Work out the finished part from the listing and answer in its coordinate system (mm). Face numbers are marked on the shaded views. A direction names the side the tool comes from. Coordinates: 2 decimals unless noted, no trailing zeros. Loops run counter-clockwise (first coordinate to the right, second up) from the corner with the lowest first, then second, coordinate; pieces in that order, holes last. Notation, with made-up numbers: (83.5, 13) -> (134.5, 13) arc R19 ccw to (134.5, 19) -> close; hole circle Ø8 at (58.5, -36). An arc over 180 degrees is marked (long way). One line per question, with ' | ' between items.
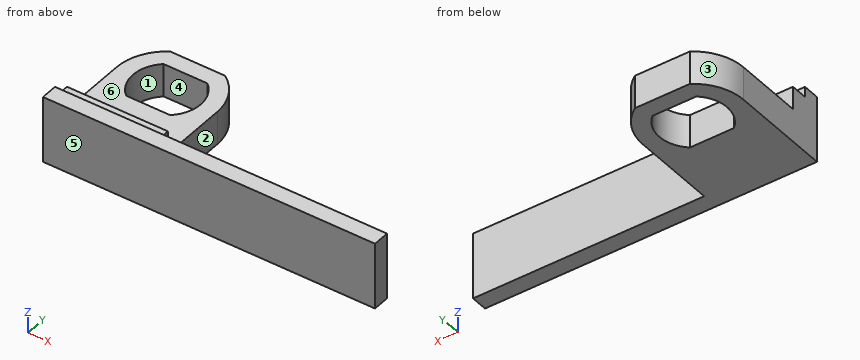
Autodesk Inventor part; units mm, degrees
ref_plane "Work Plane1" through (31.1962, 56.4165, 110.8343) normal (0, 0, 1) x (1, 0, 0)
ref_plane "Work Plane2" through (-8.5806, 30.9168, 125.8343) normal (0, 0, 1) x (1, 0, 0)
ref_plane "YZ Plane" through (0, 0, 0) normal (1, 0, 0) x (0, 1, 0)
ref_plane "Work Plane1" through (31.1962, 56.4165, 110.8343) normal (0, 0, 1) x (1, 0, 0)
sketch "Sketch2" plane through (31.1962, 56.4165, 110.8343) normal (0, 0, 1) x (1, 0, 0)
  line L0 (6.5, -7.5) -> (-6.5, -7.5) construction
  line L1 (-6.5, 7.5) -> (6.5, 7.5) construction
  arc A0 (6.5, -7.5) -> (6.5, 7.5) centre (-0.1144, 0) ccw construction
  arc A1 (-6.5, 7.5) -> (-6.5, -7.5) centre (0.1144, 0) ccw construction
  line L2 (6.6124, 7.8) -> (-6.6124, 7.8)
  arc A2 (-6.6124, 7.8) -> (-6.6124, -7.8) centre (0.1144, 0) ccw
  line L3 (-6.6124, -7.8) -> (6.6124, -7.8)
  arc A3 (6.6124, -7.8) -> (6.6124, 7.8) centre (-0.1144, 0) ccw
  line L4 (8.2671, 12.8) -> (-8.2671, 12.8)
  arc A4 (-8.2671, 12.8) -> (-8.2671, -12.8) centre (0.1144, 0) ccw
  line L5 (-8.2671, -12.8) -> (8.2671, -12.8)
  arc A5 (8.2671, -12.8) -> (8.2671, 12.8) centre (-0.1144, 0) ccw
  line L6 (15.1856, 0) -> (-15.1856, 0) construction
  line L7 (-15.1856, 0) -> (-15.1856, -30.6)
  line L8 (-15.1856, -30.6) -> (15.1856, -30.6)
  line L9 (15.1856, -30.6) -> (15.1856, 0)
  line L10 (15.1856, -30.6) -> (-15.1856, -30.6)
  line L11 (-15.1856, -30.6) -> (-15.1856, -25.6)
  line L12 (15.1856, -25.6) -> (15.1856, -30.6)
  line L13 (15.1856, -20.6) -> (-15.1856, -20.6)
  line L14 (-15.1856, -30.6) -> (84.8144, -30.6)
  line L15 (84.8144, -30.6) -> (84.8144, -25.6)
  line L16 (84.8144, -25.6) -> (-15.1856, -25.6)
  line L17 (-15.1856, -25.6) -> (-15.1856, -30.6)
  point P0 (-31.1962, -56.4165)
  point P1 (-15.1856, 0)
  dimension "d5" = 0.3
  dimension "d6" = 5
  dimension "d7" = 30.6
  dimension "d16" = 100
extrude "Extrusion1" add sketch "Sketch2" against normal blind 10 contours A5 L5 A4 L4 | L9 L13 L7 A4 L5 A5 | L9 L16 L7 L13 | L9 L8 L7 L16
ref_plane "Work Plane2" through (-8.5806, 30.9168, 125.8343) normal (0, 0, 1) x (1, 0, 0)
extrude "Extrusion2" add sketch "Sketch2" along normal blind 10 and the other way blind 10 contours L16 L15 L14 L9 | L9 L8 L7 L16
extrude "Extrusion3" add sketch "Sketch2" along normal blind 6.9 contours L9 L16 L7 L13 | L9 L8 L7 L16
properties part number "tempHolder"
1) Find section D-D (z = 103.25). Write down the section's boundary in (x, y), plus the area to 3 significant figures.
Check values:
outline: (16.01, 25.82) -> (116.01, 25.82) -> (116.01, 30.82) -> (46.38, 30.82) -> (46.38, 56.42) arc R15.3 ccw to (39.46, 69.22) -> (22.93, 69.22) arc R15.3 ccw to (16.01, 56.42) -> close; hole (24.58, 48.62) -> (37.81, 48.62) arc R10.3 ccw to (37.81, 64.22) -> (24.58, 64.22) arc R10.3 ccw to start | area: 1,330 mm^2
2) Find section B-B (y = 52.5). Write down the section's boundary in (x, z).
Check values:
outline: (16.01, 100.83) -> (21.78, 100.83) -> (21.78, 110.83) -> (16.01, 110.83) -> close; (40.61, 100.83) -> (46.38, 100.83) -> (46.38, 110.83) -> (40.61, 110.83) -> close
3) For the marked faces 1, 2 and 3, determine the directions among +Z, -Z, +X, -X, +Y, -Y from which every point of the face is accessible in a straight line to the end or side of a thin tool.
Check values:
face 1: +Z, -Z | face 2: +Z, -Z, +X, +Y | face 3: +Z, -Z, -X, +Y
4) Find section A-A (x = 26.5). Write down the section's boundary in (y, z), plus the area to 4 significant figures.
Check values:
outline: (25.82, 100.83) -> (48.62, 100.83) -> (48.62, 110.83) -> (35.82, 110.83) -> (35.82, 117.73) -> (30.82, 117.73) -> (30.82, 120.83) -> (25.82, 120.83) -> close; (64.22, 100.83) -> (69.22, 100.83) -> (69.22, 110.83) -> (64.22, 110.83) -> close | area: 362.5 mm^2
5) Find the intervals of material crossed by line 1 along Y through (x, z) = (73, 120); line 2 along Z through (x, y) = (34, 46); line 3 along Y through (x, z) = (38, 114.25), in increasing order.
Check values:
line 1: y = 25.82 to 30.82 | line 2: z = 100.83 to 110.83 | line 3: y = 25.82 to 35.82
6) Flat-ended cylindrical pins translate along their axes: pin 1 (2.5 mm diameter, centred on x = 26, y = 33, fed in from +Z); pin 2 (2 mm diameter, centred on y = 63.5, z = 109, fed in from +X); pin 3 (7.5 mm diameter, centred on x = 38, z = 115.5, fed in from +Y); pin 4 (4 mm diameter, centred on y = 57.5, z = 114.5, fed in from +X). Find the tip coordinate at first contact, or state that the pin passes through.
Check values:
pin 1: stops at z = 117.73 | pin 2: stops at x = 45.12 | pin 3: stops at y = 35.82 | pin 4: passes through
7) The mould has two halves that part along Y. Classify the marked faces 4, 5 and 6: released by +Y, released by -Y, zero draft, split by the parting line, or undercut.
Check values:
face 4: undercut | face 5: released by -Y | face 6: zero draft
8) Find section C-C (z = 115.75). Write down the section's boundary in (x, y), plus the area to 3 significant figures.
Check values:
outline: (16.01, 25.82) -> (116.01, 25.82) -> (116.01, 30.82) -> (46.38, 30.82) -> (46.38, 35.82) -> (16.01, 35.82) -> close | area: 652 mm^2
